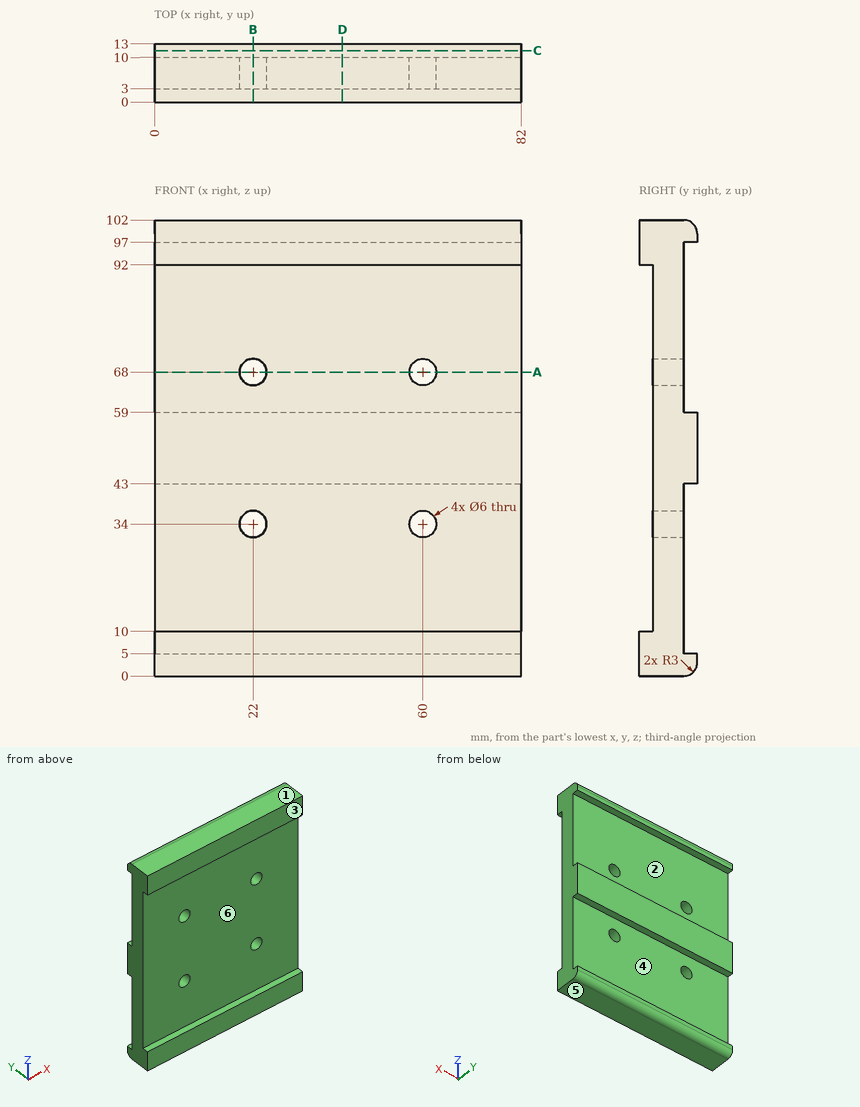
Here's the drawing with two shaded views (mm, measured from the low corner). I have some questions. A direction names the side the tool comes from. Coordinates: 2 decimals unless noted, no trailing zeros. Loops run counter-clockwise (first coordinate to the right, second up) from the corner with the lowest first, then second, coordinate; pieces in that order, holes last. Notation, with made-up numbers: (29.25, 3) -> (63.25, 3) arc R18 cw to (63.25, 28) -> close; hole circle Ø2 at (88, 82). An arc over 180 degrees is marked (long way). Put each result on its own line as item: value. Start each with the question number.
Q1. I want a section at B-B (x = 22). Write out the boundary of the cut face in (y, z).
Q2. For the marked faces 4, 5 and 6, which set-ups out of +Z, -Z, +X, -X, +Y, -Y let a thin tool reach every point of the face, with its end or its side?
Q3. I want a section at D-D (x = 42). Write out the boundary of the cut face in (y, z), plus the area to 3 significant figures.
Q4. Thinking about a two-plate mould opening in Z: for the marked faces 1, 2 and 3, which applies, pulls with the +Z half, pulls with the -Z half, needs draft (parallel to the pull), parting line crosses it, or undercut?
Q5. I'm going to push flat-ended pins straight in: P1, Ø2, axis at y = 1.5, z = 38, coming from the +X side; P2, Ø24.5, axis at x = 40.5, z = 69.5, coming from the -Y side; P3, Ø2.5, axis at x = 37, y = 12, coming from the -Z side; P4, Ø8, axis at x = 22, z = 34, coming from the +Y side. Where does each tip first touch, or does it pass through?
Q6. If I drill on line 1 (Z direction, x = 60, y = 6); line 2 (Z direction, x = 61, y = 2.5); line 3 (Y direction, x = 38, z = 76.5), over which ranges is the centre line in solid material (lowest first)? Write a range as [from, to].
Q7. I want a section at A-A (z = 68). Write out the boundary of the cut face in (x, y), plus the area to 3 significant figures.
Q8. I want a section at C-C (y = 11.5). Write out the boundary of the cut face in (x, z).
Taken from the geometry:
1. outline: (0, 0) -> (10, 0) arc R3 ccw to (13, 3) -> (13, 5) -> (10, 5) -> (10, 31) -> (3, 31) -> (3, 10) -> (0, 10) -> close; (0, 92) -> (3, 92) -> (3, 71) -> (10, 71) -> (10, 97) -> (13, 97) -> (13, 99) arc R3 ccw to (10, 102) -> (0, 102) -> close; (3, 37) -> (10, 37) -> (10, 43) -> (13, 43) -> (13, 59) -> (10, 59) -> (10, 65) -> (3, 65) -> close
2. face 4: +X, -X, +Y
2. face 5: -Z, +X, -X, +Y, -Y
2. face 6: +X, -X, -Y
3. outline: (0, 0) -> (10, 0) arc R3 ccw to (13, 3) -> (13, 5) -> (10, 5) -> (10, 43) -> (13, 43) -> (13, 59) -> (10, 59) -> (10, 97) -> (13, 97) -> (13, 99) arc R3 ccw to (10, 102) -> (0, 102) -> (0, 92) -> (3, 92) -> (3, 10) -> (0, 10) -> close
3. area: 848 mm2
4. face 1: pulls with the +Z half
4. face 2: undercut
4. face 3: needs draft
5. P1: passes through
5. P2: stops at y = 3
5. P3: stops at z = 0.1
5. P4: stops at y = 10
6. line 1: z = [0, 31], [37, 65], [71, 102]
6. line 2: z = [0, 10], [92, 102]
6. line 3: y = [3, 10]
7. outline: (0, 3) -> (19, 3) -> (19, 10) -> (0, 10) -> close; (25, 3) -> (57, 3) -> (57, 10) -> (25, 10) -> close; (63, 3) -> (82, 3) -> (82, 10) -> (63, 10) -> close
7. area: 490 mm2
8. outline: (0, 0.4) -> (82, 0.4) -> (82, 5) -> (0, 5) -> close; (0, 43) -> (82, 43) -> (82, 59) -> (0, 59) -> close; (0, 97) -> (82, 97) -> (82, 101.6) -> (0, 101.6) -> close
